Geometry: see drawing. Coordinates: mm, zero at the bounding-box minimum. A direction names the side the tool comes from. Coordinates: 2 decimals unless noted, no trailing zeros. Write each loop counter-clockwise with the first axis right and the second up, starting at its lowest first coordinate (ties: lowest second). Pieces come first, ordered by that corner, then holes.
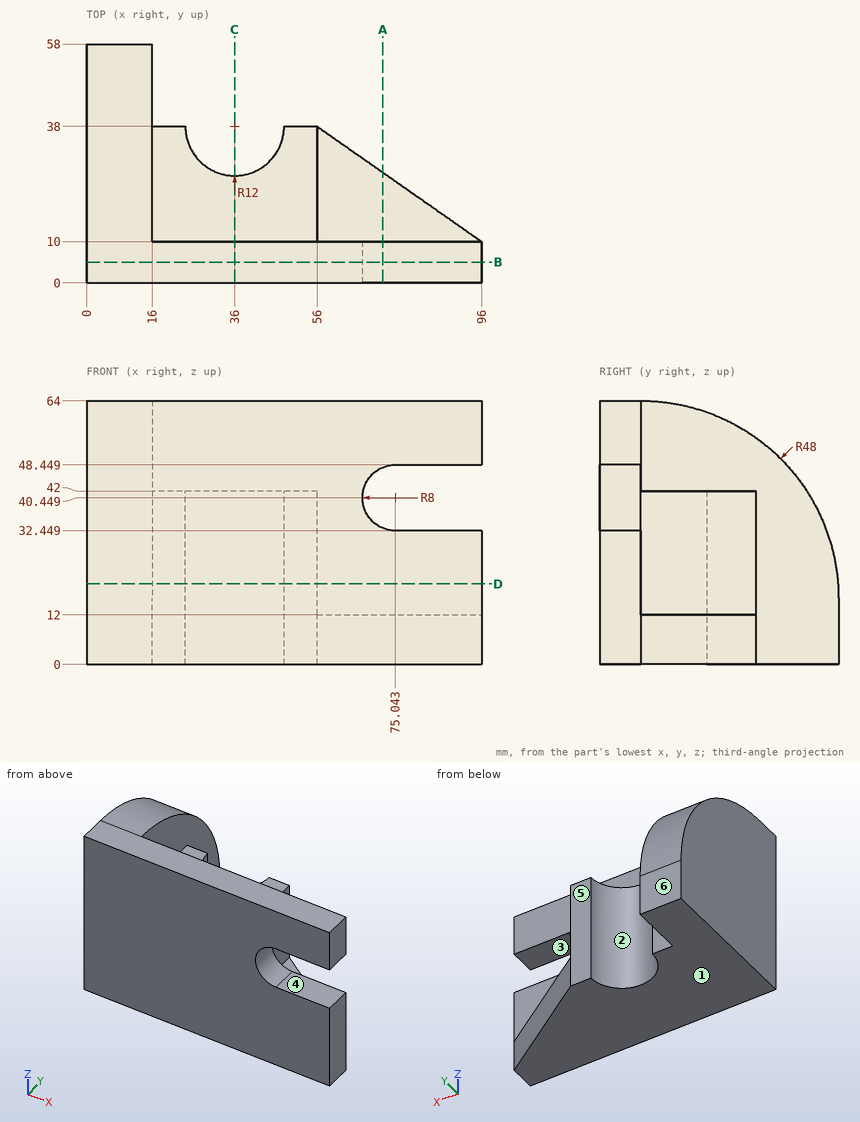
Item 1: Pin query (flat end, axial travel): pin 1 (9 mm diameter, centred on x = 50.5, z = 19.5, fed in from +Y); pin 2 (4 mm diameter, centred on x = 37.5, y = 21, fed in from +Z); pin 3 (14.5 mm diameter, centred on y = 27, z = 26.5, fed in from +X). Return the tip coordinate at first contact, or that it passes through.
Derived:
pin 1: stops at y = 38
pin 2: stops at z = 42
pin 3: stops at x = 56
Item 2: Section C-C, the plane x = 36. Output: boundary loops of the cut face in (y, z), plus the area to 3 significant figures.
Derived:
outline: (0, 0) - (26, 0) - (26, 42) - (10, 42) - (10, 64) - (0, 64) - close
area: 1,310 mm2
Item 3: Set-up query: the marked faces 4, 5 and 6. Return all of +Z, -Z, +X, -X, +Y, -Y with unobstructed straight access to the full face (end or side cutting, diameter ignored); none if empty.
Derived:
face 4: +X, +Y, -Y
face 5: +Z, -Z, +X, +Y
face 6: +Z, -Z, +X, -X, +Y
Item 4: Material intervals for probe 1 along Y at (x, z) = (80, 54); probe 2 along Z at (x, y) = (66, 16); probe 3 along X at (y, z) = (53, 19.5), sorted ascending.
Derived:
probe 1: y = 0 to 10
probe 2: z = 0 to 12
probe 3: x = 0 to 16
Item 5: Section D-D, the plane z = 19.5. Output: boundary loops of the cut face in (x, y), plus the area to 3 significant figures.
Derived:
outline: (0, 0) - (96, 0) - (96, 10) - (56, 10) - (56, 38) - (48, 38) arc R12 cw to (24, 38) - (16, 38) - (16, 57.87) - (0, 57.87) - close
area: 2,620 mm2
Item 6: Pull-direction query (Z, two-part tool) for the marked faces 1, 2 and 3; classes: released by +Z, released by -Z, zero draft, split by the parting line, or undercut.
Derived:
face 1: released by -Z
face 2: zero draft
face 3: undercut
Item 7: Section B-B, the plane y = 5. Output: boundary loops of the cut face in (x, z).
Derived:
outline: (0, 0) - (96, 0) - (96, 32.45) - (75.04, 32.45) arc R8 cw to (75.04, 48.45) - (96, 48.45) - (96, 64) - (0, 64) - close
Item 8: Section A-A, the plane x = 72. Output: boundary loops of the cut face in (y, z).
Derived:
outline: (0, 0) - (26.8, 0) - (26.8, 12) - (10, 12) - (10, 33.05) - (0, 33.05) - close; (0, 47.85) - (10, 47.85) - (10, 64) - (0, 64) - close
